The model under review builds one solid part; all positions refer to its coordinate system, in mm. A direction names the side the tool comes from. Coordinates: 2 decimals unless noted, no trailing zeros. Order: outer loops, then holes, each group sorted by start corner. A loop starts at its lowest first (then second) coordinate and runs counter-clockwise, first axis right, second up. Notation, with made-up numbers: (-17.5, 1.25) -> (41.5, 1.25) arc R22 cw to (41.5, 29.25) -> close; hole circle Ø8 at (-28, 32.5). An arc over 180 degrees is marked (long way). Use CSV: the item, a comma, the result in double quotes. Start each with the question number.
```python
from build123d import *

# Parameters (mm, degrees)
SKETCH1_R           = 6
SKETCH1_R_2         = 1.5
BOSS_EXTRUDE1_DEPTH = 3.175


with BuildPart() as part:
    # Sketch1 → Boss-Extrude1 (new body)
    with BuildSketch(Plane.XY):
        Polygon((18.5, 0), (18.5, -3.175), (0, -3.175), (0, 0), (0, 37), (37, 37), (37, 0), align=None)
        with Locations((18.39023312, 12.089873912)):
            Circle(SKETCH1_R, mode=Mode.SUBTRACT)
        with Locations((2.89023312, 19.089873912)):
            Circle(SKETCH1_R_2, mode=Mode.SUBTRACT)
        with Locations((10.64023312, 5.666480153)):
            Circle(SKETCH1_R_2, mode=Mode.SUBTRACT)
        with Locations((26.14023312, 5.666480153)):
            Circle(SKETCH1_R_2, mode=Mode.SUBTRACT)
        with Locations((33.89023312, 19.089873912)):
            Circle(SKETCH1_R_2, mode=Mode.SUBTRACT)
        with Locations((26.14023312, 32.513267671)):
            Circle(SKETCH1_R_2, mode=Mode.SUBTRACT)
        with Locations((10.64023312, 32.513267671)):
            Circle(SKETCH1_R_2, mode=Mode.SUBTRACT)
    extrude(amount=BOSS_EXTRUDE1_DEPTH)


solid = part.part
```
Q1. For faces 4 (the flat face through (28, 0, 2)), 5 (the cylindrical face through (25.945, 7.154, 1.565)), list the 3-axis set-ups (+Z, -Z, +X, -X, +Y, -Y) from which the entire face can be reached by the end or side of a thin tool; tool diameter is ignored.
Q2. Draft analysis for pull direction X (two halves, no side actions). For faces 1 (the flat face through (9, -3.175, 2)), 2 (the cylindrical face through (11.45, 6.93, 1.57)), 3 (the flat face through (18.5, -2, 2)), state which applies: +X half, -X half, draft (parallel to the pull), parting line (faces both ways), or undercut.
Q3. Add section A-A, the plane y = 13. State the section outline as (x, z) points (3 decimals).
Q4. Clearance check with a flat-ended pin moving along its axis: pin 1 Ø1.6 at (y, z) = (-1.5, 1.5) entering from +X. State where the tip first meets the part, or that it passes through.
Q5. To check wall thickness, follow probe 1 along Y at (x, z) = (9.5, 1.8) (3 decimals); probe 2 along X at (y, z) = (6, 0.45); probe 3 along X at (y, z) = (19, 2.3). State the ranges of each line that lie inside material, in increasing order.
Q6. Add section C-C, the plane x = 31. State the section outline as (y, z) points (3 decimals), then the cut area to 3 significant figures.
Q7. Add section D-D, the plane y = 31.5. State the section outline as (x, z) points (3 decimals).
Q8. Add section B-B, the plane z = 0.8. State the section outline as (x, y) points (3 decimals), then the cut area to 3 significant figures.
Answer block:
1,face 4,"+Z, -Z, +X, -Y"
1,face 5,"+Z, -Z"
2,face 1,"draft"
2,face 2,"undercut"
2,face 3,"+X half"
3,outline,"(0, 0) -> (12.46, 0) -> (12.46, 3.175) -> (0, 3.175) -> close; (24.321, 0) -> (37, 0) -> (37, 3.175) -> (24.321, 3.175) -> close"
4,pin 1,"stops at x = 18.5"
5,probe 1,"y = -3.175 to 4.692, 6.641 to 31.539, 33.488 to 37"
5,probe 2,"x = 0 to 9.18, 12.1 to 24.68, 27.6 to 37"
5,probe 3,"x = 0 to 1.39, 4.39 to 32.39, 35.39 to 37"
6,outline,"(0, 0) -> (37, 0) -> (37, 3.175) -> (0, 3.175) -> close"
6,area,"117 mm²"
7,outline,"(0, 0) -> (9.534, 0) -> (9.534, 3.175) -> (0, 3.175) -> close; (11.746, 0) -> (25.034, 0) -> (25.034, 3.175) -> (11.746, 3.175) -> close; (27.246, 0) -> (37, 0) -> (37, 3.175) -> (27.246, 3.175) -> close"
8,outline,"(0, -3.175) -> (18.5, -3.175) -> (18.5, 0) -> (37, 0) -> (37, 37) -> (0, 37) -> close; hole circle Ø3 at (2.89, 19.09); hole circle Ø3 at (10.64, 5.666); hole circle Ø3 at (10.64, 32.513); hole circle Ø12 at (18.39, 12.09); hole circle Ø3 at (26.14, 5.666); hole circle Ø3 at (26.14, 32.513); hole circle Ø3 at (33.89, 19.09)"
8,area,"1,270 mm²"
